For this review, take the finished solid that the model builds, in its own axes (mm). A direction names the side the tool comes from. Round coordinates to 2 decimals unless told otherwise and drop trailing zeros. Loops run counter-clockwise (first coordinate to the right, second up) from the corner with the lowest first, then second, coordinate; pieces in that order, holes last.
1. Consider section A-A on z = 10.75. State the section outline as (x, y) points, then the cut area to 3 significant figures.
2. Consider section C-C on z = 6.25. State the section outline as (x, y) points.
3. Clearance check with flat-ended pins moving along their axes: pin 1 Ø1.5 at (x, y) = (-2.5, 24) entering from -Z; pin 2 Ø4 at (x, y) = (19, 4.5) entering from -Z. State where each tip first meets the part, or that it passes through.
4. Consider section B-B on x = 7. State the section outline as (y, z) points, then the cut area to 3 significant figures.
5. Tool access review of faces 5 (the flat face through (0, 22, 10)), 6 (the flat face through (-2.15, 0, 13)), 7 (the flat face through (-24, -17.5, 4)), 8 (the flat face through (17.5, 23, 4)), 9 (the flat face through (-25, 0, 11)): name each direction out of +Z, -Z, +X, -X, +Y, -Y from which nothing blocks a thin tool from reaching the whole face with its end or side.
6. To check wall thickness, follow line 1 along Y through (x, z) = (17.5, 9.5); line 2 along Z through (x, y) = (-10, -14); line 3 along Z through (x, y) = (1, 23.5). State the ranges of each line that lie inside material, in increasing order.
7. Draft analysis for pull direction Y (two halves, no side actions). For faces 1 (the flat face through (22, 23, 0)), 2 (the flat face through (23, 0, 9)), 3 (the flat face through (0, 25, 11)), 4 (the flat face through (24, 17.5, 4)), state which applies: released by +Y, released by -Y, zero draft, split by the parting line, or undercut.
from build123d import *

# Parameters (mm, degrees)
SKETCH1_W               = 50
SKETCH1_H               = 50
BOSS_EXTRUDE1_DEPTH     = 15
SHELL1_T                = -3
CUT_EXTRUDE1_DEPTH      = 1
CUT_EXTRUDE1_DEPTH_BACK = 16
CUT_EXTRUDE2_DEPTH      = 9


with BuildPart() as part:
    # Sketch1 → Boss-Extrude1 (new body)
    with BuildSketch(Plane.XY):
        Rectangle(SKETCH1_W, SKETCH1_H)
    extrude(amount=BOSS_EXTRUDE1_DEPTH)

    # Shell1
    shell1_openings = [part.faces().sort_by_distance(p)[0] for p in [
        (0, 0, 0),
    ]]
    offset(amount=SHELL1_T, openings=shell1_openings, kind=Kind.INTERSECTION)

    # Sketch2 → Cut-Extrude1 (cut, two sides)
    with BuildSketch(Plane(origin=(0, 0, 0), x_dir=(-1, 0, 0), z_dir=(0, 0, -1))) as cut_extrude1_sk:
        with BuildLine():
            Line((-2.15, 1.37113092), (-2.15, -1.37113092))
            ThreePointArc((-2.15, -1.37113092), (0, -2.55), (2.15, -1.37113092))
            Line((2.15, -1.37113092), (2.15, 1.37113092))
            ThreePointArc((2.15, 1.37113092), (0, 2.55), (-2.15, 1.37113092))
        make_face()
    extrude(amount=CUT_EXTRUDE1_DEPTH, mode=Mode.SUBTRACT)
    extrude(cut_extrude1_sk.sketch, amount=-CUT_EXTRUDE1_DEPTH_BACK, mode=Mode.SUBTRACT)

    # Sketch4 → Cut-Extrude2 (cut)
    with BuildSketch(Plane(origin=(0, 0, 0), x_dir=(-1, 0, 0), z_dir=(0, 0, -1))):
        Polygon((-17.5, 17.5), (-17.5, 27.948399717), (17.5, 27.948399717), (17.5, 17.5), (26.941451912, 17.5), (26.941451912, -17.5), (17.5, -17.5), (17.5, -27.948399717), (-17.5, -27.948399717), (-17.5, -17.5), (-26.941451912, -17.5), (-26.941451912, 17.5), align=None)
    extrude(amount=-CUT_EXTRUDE2_DEPTH, mode=Mode.SUBTRACT)


solid = part.part
Resolved:
1. outline: (-25, -25) - (25, -25) - (25, 25) - (-25, 25) - close; hole (-22, -22) - (22, -22) - (22, 22) - (-22, 22) - close
1. area: 564 mm2
2. outline: (-25, -25) - (-17.5, -25) - (-17.5, -22) - (-22, -22) - (-22, -17.5) - (-25, -17.5) - close; (-25, 17.5) - (-22, 17.5) - (-22, 22) - (-17.5, 22) - (-17.5, 25) - (-25, 25) - close; (17.5, -25) - (25, -25) - (25, -17.5) - (22, -17.5) - (22, -22) - (17.5, -22) - close; (17.5, 22) - (22, 22) - (22, 17.5) - (25, 17.5) - (25, 25) - (17.5, 25) - close
3. pin 1: stops at z = 9
3. pin 2: stops at z = 12
4. outline: (-25, 9) - (-22, 9) - (-22, 12) - (22, 12) - (22, 9) - (25, 9) - (25, 15) - (-25, 15) - close
4. area: 168 mm2
5. face 5: -Z
5. face 6: +Z, -Z
5. face 7: -Z, +X, -X
5. face 8: -Z, +Y, -Y
5. face 9: +Z, -Z, -X, +Y, -Y
6. line 1: y = -25 to -22, 22 to 25
6. line 2: z = 12 to 15
6. line 3: z = 9 to 15
7. face 1: zero draft
7. face 2: undercut
7. face 3: released by +Y
7. face 4: undercut
